Check sheet for the modelled part. Datum: model origin and axes. Units: mm. A direction names the side the tool comes from. Coordinates: 2 decimals unless noted, no trailing zeros. Loops run counter-clockwise (first coordinate to the right, second up) from the corner with the lowest first, then second, coordinate; pieces in that order, holes last. Notation, with made-up numbers: M 67.5,50.25 L 108.5,50.25 A12 cw 108.5,73.25 Z; hole C 59,77 d1. An arc over 180 degrees is marked long. Use CSV: the item, a comma, the result in double quotes. Start each with the question number.
(1) Draft check along Y on faces 4 (the flat face through (-9, 4, 8)), 5 (the flat face through (-12, 6.6, 8)). Enter one of: pulls with the +Y half, pulls with the -Y half, needs draft (parallel to the pull), parting line crosses it, or undercut.
(2) Section check D-D on z = 10.25. Record the cut outline in (x, y).
(3) Set-up check for faces 1 (the flat face through (-22, 6.6, 8)), 2 (the flat face through (-20.7, 4.1, 9.2)), 3 (the flat face through (-17, 4, 4)): record each of +Z, -Z, +X, -X, +Y, -Y from which the full face is reachable in a straight line by a thin tool's end or side.
(4) Go/stop test with flat-tipped pins: pin 1 Ø0.8 at (x, y) = (-23, 7.5) entering from +Z; pin 2 Ø3 at (x, y) = (-13, 7.5) entering from +Z. Record where each tip stops, or that it passes through.
(5) Section check C-C on x = -11. Record the cut outline in (y, z).
(6) Section check B-B on y = 8. Record the cut outline in (x, z), and give its area (4 significant figures).
(7) Scan lines: line 1 (Y direction, x = -12.5, z = 8.75); line 2 (Z direction, x = -13.75, y = -0.25); line 3 (Z direction, x = -17.5, y = -2). Record each from-to range of solid material in increasing order.
(8) Section check A-A on z = 8. Record the cut outline in (x, y).
from build123d import *

# Parameters (mm, degrees)
RESSALTO_EXTRUS_O1_DEPTH  = 16
ESBO_O2_W                 = 2.8
ESBO_O2_H                 = 2.8
CORTE_EXTRUS_O1_DEPTH     = 54.103672189
ESBO_O4_W                 = 2.8
ESBO_O4_H                 = 2.8
CORTE_EXTRUS_O2_DEPTH     = 31.186917696
CORPO_MOVER_COPIAR1_ANGLE = 90
ESBO_O6_W                 = 30
ESBO_O6_H                 = 16
CORTE_EXTRUS_O3_DEPTH     = 29.861739379
ESBO_O7_W                 = 25.221413321
ESBO_O7_H                 = 12.57615678
RESSALTO_EXTRUS_O2_DEPTH  = 2.5
ESBO_O8_W                 = 2.8
ESBO_O8_H                 = 2.8
CORTE_EXTRUS_O4_DEPTH     = 29.271009886
ESBO_O10_W                = 32
ESBO_O10_H                = 16
CORTE_EXTRUS_O5_DEPTH     = 10


with BuildPart() as part:
    # Esboço1 → Ressalto-extrusão1 (new body)
    with BuildSketch(Plane.XY):
        Polygon((-25, 0), (25, 0), (25, 8), (23.5, 8), (18, 2.5), (-18, 2.5), (-23.5, 8), (-25, 8), align=None)
    extrude(amount=RESSALTO_EXTRUS_O1_DEPTH)

    # Esboço2 → Corte-extrusão1 (cut, through all)
    with BuildSketch(Plane(origin=(25, 0, 0), x_dir=(0, 0, -1), z_dir=(1, 0, 0))):
        with Locations((-4, 4)):
            Rectangle(ESBO_O2_W, ESBO_O2_H)
        with Locations((-12, 4)):
            Rectangle(ESBO_O2_W, ESBO_O2_H)
    extrude(amount=-CORTE_EXTRUS_O1_DEPTH, mode=Mode.SUBTRACT)

    # Esboço4 → Corte-extrusão2 (cut, through all)
    with BuildSketch(Plane(origin=(0, 2.5, 0), x_dir=(1, 0, 0), z_dir=(0, 1, 0))):
        with Locations((-16, -4)):
            Rectangle(ESBO_O4_W, ESBO_O4_H)
        with Locations((-8, -4)):
            Rectangle(ESBO_O4_W, ESBO_O4_H)
        with Locations((0, -4)):
            Rectangle(ESBO_O4_W, ESBO_O4_H)
        with Locations((8, -4)):
            Rectangle(ESBO_O4_W, ESBO_O4_H)
        with Locations((16, -4)):
            Rectangle(ESBO_O4_W, ESBO_O4_H)
        with Locations((-8, -12)):
            Rectangle(ESBO_O4_W, ESBO_O4_H)
        with Locations((0, -12)):
            Rectangle(ESBO_O4_W, ESBO_O4_H)
        with Locations((8, -12)):
            Rectangle(ESBO_O4_W, ESBO_O4_H)
        with Locations((16, -12)):
            Rectangle(ESBO_O4_W, ESBO_O4_H)
        with Locations((-16, -12)):
            Rectangle(ESBO_O4_W, ESBO_O4_H)
    extrude(amount=-CORTE_EXTRUS_O2_DEPTH, mode=Mode.SUBTRACT)


with BuildPart() as part_1:
    # Corpo-Mover/Copiar1: moved
    add(part.part.rotate(Axis((0, 4, 8), (1, 0, 0)), CORPO_MOVER_COPIAR1_ANGLE))

    # Esboço6 → Corte-extrusão3 (cut, through all)
    with BuildSketch(Plane(origin=(0, 0, 4), x_dir=(-1, 0, 0), z_dir=(0, 0, -1))):
        with Locations((-10, 4)):
            Rectangle(ESBO_O6_W, ESBO_O6_H)
    extrude(amount=-CORTE_EXTRUS_O3_DEPTH, mode=Mode.SUBTRACT)

    # Espelhar3: part across plane


with BuildPart() as part_2:
    add(part_1.part)
    add(part_1.part.mirror(Plane(origin=(-5, -4, 12), x_dir=(0, 0, 1), z_dir=(-1, 0, 0))))

    # Esboço7 → Ressalto-extrusão2 (add, through all)
    with BuildSketch(Plane.XY.offset(6.5)):
        with Locations((-4.971284079, 3.626460754)):
            Rectangle(ESBO_O7_W, ESBO_O7_H)
    extrude(amount=-RESSALTO_EXTRUS_O2_DEPTH)

    # Esboço8 → Corte-extrusão4 (cut, through all)
    with BuildSketch(Plane.XY.offset(6.5)):
        with Locations((-5, 8)):
            Rectangle(ESBO_O8_W, ESBO_O8_H)
        with Locations((-13, 8)):
            Rectangle(ESBO_O8_W, ESBO_O8_H)
        with Locations((3, 8)):
            Rectangle(ESBO_O8_W, ESBO_O8_H)
        with Locations((-5, 0)):
            Rectangle(ESBO_O8_W, ESBO_O8_H)
        with Locations((3, 0)):
            Rectangle(ESBO_O8_W, ESBO_O8_H)
        with Locations((-13, 0)):
            Rectangle(ESBO_O8_W, ESBO_O8_H)
    extrude(amount=-CORTE_EXTRUS_O4_DEPTH, mode=Mode.SUBTRACT)

    # Esboço10 → Corte-extrusão5 (cut)
    with BuildSketch(Plane(origin=(0, 0, 4), x_dir=(-1, 0, 0), z_dir=(0, 0, -1))):
        with Locations((1, 4)):
            Rectangle(ESBO_O10_W, ESBO_O10_H)
    extrude(amount=-CORTE_EXTRUS_O5_DEPTH, mode=Mode.SUBTRACT)

    # Espelhar4: part across plane


with BuildPart() as part_3:
    add(part_2.part)
    add(part_2.part.mirror(Plane(origin=(-17, -4, 14), x_dir=(0, 0, 1), z_dir=(-1, 0, 0))))


solid = part_3.part
Outcome:
1,face 4,"needs draft"
1,face 5,"undercut"
2,outline,"M -25,-4 L -21.75,-4 L -21.75,12 L -25,12 Z; M -12.25,-4 L -9,-4 L -9,12 L -12.25,12 Z"
3,face 1,"+X, -X"
3,face 2,"+Z, +Y, -Y"
3,face 3,"-Z, +X, -X, +Y, -Y"
4,pin 1,"stops at z = 11.9"
4,pin 2,"stops at z = 11"
5,outline,"M -4,4 L 12,4 L 12,11.5 L -4,11.5 Z; hole M -1.4,6.6 L 1.4,6.6 L 1.4,9.4 L -1.4,9.4 Z; hole M 6.6,6.6 L 9.4,6.6 L 9.4,9.4 L 6.6,9.4 Z"
6,outline,"M -25,4 L -9,4 L -9,6.6 L -15.9,6.6 L -16,6.5 L -18,6.5 L -18.1,6.6 L -25,6.6 Z; M -25,9.4 L -20.9,9.4 L -23.5,12 L -25,12 Z; M -13.1,9.4 L -9,9.4 L -9,12 L -10.5,12 Z"
6,area,"55.95 mm²"
7,line 1,"y = -4 to -1.4, 1.4 to 6.6, 9.4 to 12"
7,line 2,"z = 4 to 6.6"
7,line 3,"z = 4 to 6.5"
8,outline,"M -25,-4 L -19.5,-4 L -19.5,-1.4 L -25,-1.4 Z; M -25,1.4 L -19.5,1.4 L -19.5,6.6 L -25,6.6 Z; M -25,9.4 L -19.5,9.4 L -19.5,12 L -25,12 Z; M -14.5,-4 L -9,-4 L -9,-1.4 L -14.5,-1.4 Z; M -14.5,1.4 L -9,1.4 L -9,6.6 L -14.5,6.6 Z; M -14.5,9.4 L -9,9.4 L -9,12 L -14.5,12 Z"
